Autodesk Fusion 360 part; units mm, degrees
sketch "Sketch1" plane through (0, 0, 0) normal (0, 1, 0) x (1, 0, 0)
  line L0 (0, 0) -> (22, 0)
  line L1 (22, 0) -> (22, -13.5)
  line L2 (22, -13.5) -> (0, -13.5)
  line L3 (0, -13.5) -> (0, 0)
  line L4 (0, -3.5) -> (22, -3.5)
  line L5 (0, -8.5) -> (22, -8.5) construction
  circle A0 centre (4.6, -8.5) radius 1.55
  circle A1 centre (17.5, -8.5) radius 1.55
  dimension "d1" = 22
  dimension "d2" = 13.5
  dimension "d3" = 3.5
  dimension "d4" = 5
  dimension "d5" = 3.1
  dimension "d6" = 3.1
  dimension "d7" = 12.9
  dimension "d8" = 4.5
extrude "Extrude1" add sketch "Sketch1" along normal blind 3.5 contours L1 L2 L3 L4
extrude "Extrude2" add sketch "Sketch1" along normal blind 48.4 contours L0 L1 L3 L4
sketch "Sketch2" plane through (0, 0, 0) normal (0, 0, -1) x (-1, 0, 0)
  line L0 (-22, 0) -> (0, 0)
  line L1 (0, 0) -> (0, 48.4)
  line L2 (0, 48.4) -> (-22, 48.4)
  line L3 (-22, 48.4) -> (-22, 0)
  line L4 (-22, 43.4) -> (0, 43.4) construction
  line L5 (0, 0) -> (-22, 0)
  circle A0 centre (-17.4, 43.4) radius 1.55
  circle A1 centre (-4.5, 43.4) radius 1.55
  dimension "d13" = 43.4
  dimension "d14" = 3.1
  dimension "d15" = 3.1
  dimension "d16" = 12.9
  dimension "d17" = 4.5
extrude "Extrude3" cut sketch "Sketch2" against normal up to surface (3.5 mm away) contours A0 | A1
fillet "Fillet1" radius 2 1 edges at (11, 3.5, 3.5)
Geometry check sheet. Reference: the model listing, model coordinates, mm. A direction names the side the tool comes from. Round coordinates to 2 decimals unless told otherwise and drop trailing zeros. Write each loop counter-clockwise with the first axis right and the second up, starting at its lowest first coordinate (ties: lowest second). Pieces come first, ordered by that corner, then holes. Notation, with made-up numbers: (41.25, -14) -> (100.25, -14) arc R31 cw to (100.25, 16) -> close; hole circle Ø7 at (32.25, 60.5). An arc over 180 degrees is marked (long way). Put each result on its own line as item: value.
1) Cross-section at A-A, the plane y = 43.4. Enter the section's corners in (x, z).
Recorded:
outline: (0, 0) -> (2.95, 0) -> (2.95, 3.5) -> (0, 3.5) -> close; (6.05, 0) -> (15.85, 0) -> (15.85, 3.5) -> (6.05, 3.5) -> close; (18.95, 0) -> (22, 0) -> (22, 3.5) -> (18.95, 3.5) -> close
2) Access from +Z, -Z, +X, -X, +Y, -Y to the whole of each face (thin tool, end or side, straight path). Record for faces 4 (the face through (11, 2, 13.5)), 5 (the face through (11, 27, 3.5)).
Recorded:
face 4: +Z, +X, -X, +Y, -Y
face 5: +Z, +X, -X, +Y
3) Cross-section at B-B, the plane z = 7.5. Enter the section's corners in (x, y).
Recorded:
outline: (0, 0) -> (3.42, 0) -> (3.42, 3.5) -> (0, 3.5) -> close; (5.78, 0) -> (16.32, 0) -> (16.32, 3.5) -> (5.78, 3.5) -> close; (18.68, 0) -> (22, 0) -> (22, 3.5) -> (18.68, 3.5) -> close
4) Cross-section at C-C, the plane x = 9.25. Enter the section's corners in (y, z), plus the area to 3 significant figures.
Recorded:
outline: (0, 0) -> (48.4, 0) -> (48.4, 3.5) -> (5.5, 3.5) arc R2 cw to (3.5, 5.5) -> (3.5, 13.5) -> (0, 13.5) -> close
area: 205 mm2
5) Cross-section at D-D, the plane x = 17.4. Enter the section's corners in (y, z), plus the area to 3 significant figures.
Recorded:
outline: (0, 0) -> (41.85, 0) -> (41.85, 3.5) -> (5.5, 3.5) arc R2 cw to (3.5, 5.5) -> (3.5, 6.95) -> (0, 6.95) -> close; (0, 10.05) -> (3.5, 10.05) -> (3.5, 13.5) -> (0, 13.5) -> close; (44.95, 0) -> (48.4, 0) -> (48.4, 3.5) -> (44.95, 3.5) -> close
area: 184 mm2
6) Depth check by flat-ended pin: P1, Ø4, axis at x = 17.5, z = 8.5, coming from the +Y side; P2, Ø11, axis at x = 12.5, y = 26.5, coming from the +Z side; P3, Ø6, axis at x = 13, z = 7, coming from the +Y side. Enter the tip coordinate at first touch or a pass-through.
Recorded:
P1: stops at y = 3.5
P2: stops at z = 3.5
P3: stops at y = 4.18
7) Thickness scan on probe 1 along Y at (x, z) = (17.4, 2); probe 2 along Z at (x, y) = (17.5, 2.6); probe 3 along X at (y, z) = (2.4, 8.5). Record the ranges inside material, lowest first. Write a range as from..to.
Recorded:
probe 1: y = 0..41.85, 44.95..48.4
probe 2: z = 0..6.95, 10.05..13.5
probe 3: x = 0..3.05, 6.15..15.95, 19.05..22
8) Release check for a two-part mould opening along Y. For faces 1 (the face through (11.15, 4.07, 4.1)), 2 (the face through (17.602, 44.937, 1.726)), 3 (the face through (11, 24, 0)) record: pulls with the +Y half, pulls with the -Y half, needs draft (parallel to the pull), parting line crosses it, or undercut.
Recorded:
face 1: pulls with the +Y half
face 2: undercut
face 3: needs draft
